Verification items for the finished model (mm, model axes). A direction names the side the tool comes from. Coordinates: 2 decimals unless noted, no trailing zeros. Order: outer loops, then holes, each group sorted by start corner. A loop starts at its lowest first (then second) coordinate and runs counter-clockwise, first axis right, second up. Notation, with made-up numbers: (41, 77.5) -> (81, 77.5) arc R31 ccw to (81, 113.5) -> close; hole circle Ø9 at (2.25, 0). An arc over 180 degrees is marked (long way). Use CSV: the item, a comma, the result in double quotes. Start each with the question number.
1) Tool access check on faces 1 (the flat face through (-24, -34, 0)), 2 (the flat face through (-41.776, -19, -10)), 3 (the flat face through (-27.565, -34, -10)), 4 (the flat face through (-33.537, -42, -10)). Record the directions out of +Z, -Z, +X, -X, +Y, -Y that give a thin tool (end or side, any length) a straight path to the whole face; none if there is none.
2) Release check for a two-part mould opening along Z. For faces 5 (the flat face through (-29, -20, 3.175)), 6 (the flat face through (-29, -20, -23.495)), 7 (the flat face through (-31.339, -34, -10)) record: released by +Z, released by -Z, zero draft, split by the parting line, or undercut.
3) Sectioned sample at D-D on y = -29.5. Record the boundary of the cut face in (x, z) (3 decimals), then the cut area to 3 significant figures.
4) Sectioned sample at A-A on x = -37. Record the boundary of the cut face in (y, z) (3 decimals), then the cut area to 3 significant figures.
5) Sectioned sample at C-C on y = -14. Record the boundary of the cut face in (x, z) (3 decimals).
6) Sectioned sample at B-B on z = -19.5. Record the boundary of the cut face in (x, y).
7) Scan lines: line 1 along Z through (x, y) = (-21, -27) (3 decimals); line 2 along X through (y, z) = (-36.5, -4.25); line 3 along Y through (x, z) = (-1, -12). Record each from-to range of solid material in increasing order.
8) Go/stop test with flat-tipped pins: pin 1 (1.6 mm diameter, centred on x = 4, y = -42.5, fed in from -Z); pin 2 (12 mm diameter, centred on y = -26.5, z = -16, fed in from +X); pin 3 (10 mm diameter, centred on x = -8, z = -9.5, fed in from +Y). Record where each tip stops, or that it passes through.
from build123d import *

# Parameters (mm, degrees)
BOSS_EXTRUDE1_DEPTH = 3.175
SKETCH2_W           = 13.335000012
SKETCH2_H           = 49.21889014
SKETCH2_R           = 1.75
BOSS_EXTRUDE2_DEPTH = 3.175
SKETCH3_W           = 46.34698368
SKETCH3_H           = 3.175
BOSS_EXTRUDE3_DEPTH = 10.160000012
SKETCH4_R           = 1.75
SKETCH4_R_2         = 3.05
CUT_EXTRUDE1_DEPTH  = 8.255
SKETCH5_W           = 3.773247043
SKETCH5_H           = 20.320000025
BOSS_EXTRUDE4_DEPTH = 12.954
SKETCH6_W           = 34.699402295
SKETCH6_H           = 0.254
CUT_EXTRUDE2_DEPTH  = 33.02


with BuildPart() as part:
    # Sketch1 → Boss-Extrude1 (new body)
    with BuildSketch(Plane.XY):
        Polygon((-22.541561274, 5.323288391), (-8.422284226, -43.895601749), (-38.601131181, -43.895601749), (-38.601131181, 5.323288391), align=None)
    extrude(amount=BOSS_EXTRUDE1_DEPTH)

    # Sketch2 → Boss-Extrude2 (add)
    with BuildSketch(Plane.ZY.offset(38.601131181)):
        with Locations((-3.492500006, -19.286156679)):
            Rectangle(SKETCH2_W, SKETCH2_H)
        with Locations(Location((-5.139541866, -3.179625598, 0), (0, 0, 270))):
            Circle(SKETCH2_R, mode=Mode.SUBTRACT)
        with Locations(Location((-5.139541866, -13.22054189, 0), (0, 0, 270))):
            Circle(SKETCH2_R, mode=Mode.SUBTRACT)
    extrude(amount=BOSS_EXTRUDE2_DEPTH)

    # Sketch3 → Boss-Extrude3 (add)
    with BuildSketch(Plane(origin=(0, 0, 0), x_dir=(-1, 0, 0), z_dir=(0, 0, -1))):
        with Locations((10.363026284, -42.308101749)):
            Rectangle(SKETCH3_W, SKETCH3_H)
    extrude(amount=BOSS_EXTRUDE3_DEPTH)

    # Sketch4 → Cut-Extrude1 (cut)
    with BuildSketch(Plane(origin=(0, -40.720601749, 0), x_dir=(1, 0, 0), z_dir=(0, 1, 0))):
        with Locations(Location((-3.706673055, 5.129541844, 0), (0, 0, 270))):
            Circle(SKETCH4_R)
        with Locations(Location((-23.788505641, 5.129541844, 0), (0, 0, 270))):
            Circle(SKETCH4_R)
        with Locations((6.334243237, 15.170458137)):
            Circle(SKETCH4_R)
        with Locations((-8.727131202, 10.149999991)):
            Circle(SKETCH4_R_2)
        with Locations(Location((6.334243237, 5.129541844, 0), (0, 0, 270))):
            Circle(SKETCH4_R)
        with Locations(Location((-13.747589348, 5.129541844, 0), (0, 0, 270))):
            Circle(SKETCH4_R)
        with Locations((-23.788505641, 15.170458137)):
            Circle(SKETCH4_R)
        with Locations((-3.706673055, 15.170458137)):
            Circle(SKETCH4_R)
        with Locations((-13.747589348, 15.170458137)):
            Circle(SKETCH4_R)
    extrude(amount=-CUT_EXTRUDE1_DEPTH, mode=Mode.SUBTRACT)

    # Mirror3: part across plane


with BuildPart() as part_1:
    add(part.part)
    add(part.part.mirror(Plane(origin=(-41.776131181, 5.323288391, -10.160000012), x_dir=(1, 0, 0), z_dir=(0, 0, 1))))

    # Sketch5 → Boss-Extrude4 (add)
    with BuildSketch(Plane(origin=(0, -40.720601749, 0), x_dir=(1, 0, 0), z_dir=(0, 1, 0))):
        with Locations((-29.452107965, 10.160000013)):
            Rectangle(SKETCH5_W, SKETCH5_H)
    extrude(amount=BOSS_EXTRUDE4_DEPTH)

    # Sketch6 → Cut-Extrude2 (cut)
    with BuildSketch(Plane(origin=(0, 5.323288391, 0), x_dir=(1, 0, 0), z_dir=(0, 1, 0))):
        with Locations((-21.251430034, 20.447000025)):
            Rectangle(SKETCH6_W, SKETCH6_H)
        with Locations((-21.251430034, -0.127)):
            Rectangle(SKETCH6_W, SKETCH6_H)
    extrude(amount=-CUT_EXTRUDE2_DEPTH, mode=Mode.SUBTRACT)


solid = part_1.part
Answers follow:
1,face 1,"+Y"
1,face 2,"+Z, -Z, -X, +Y, -Y"
1,face 3,"+X, +Y"
1,face 4,"+Y, -Y"
2,face 5,"released by +Z"
2,face 6,"released by -Z"
2,face 7,"undercut"
3,outline,"(-41.776, -23.495) -> (-12.552, -23.495) -> (-12.552, -20.32) -> (-27.565, -20.32) -> (-27.565, 0) -> (-12.552, 0) -> (-12.552, 3.175) -> (-41.776, 3.175) -> close; hole (-38.601, -20.32) -> (-31.339, -20.32) -> (-31.339, 0) -> (-38.601, 0) -> close"
3,area,"327 mm²"
4,outline,"(-43.896, -23.495) -> (5.323, -23.495) -> (5.323, -20.574) -> (-27.697, -20.574) -> (-27.697, -20.32) -> (-43.896, -20.32) -> close; (-43.896, 0) -> (-27.697, 0) -> (-27.697, 0.254) -> (5.323, 0.254) -> (5.323, 3.175) -> (-43.896, 3.175) -> close"
4,area,"296 mm²"
5,outline,"(-41.776, -23.495) -> (-16.998, -23.495) -> (-16.998, -20.574) -> (-38.601, -20.574) -> (-38.601, -16.747) -> (-41.776, -16.747) -> close; (-41.776, -13.614) -> (-38.601, -13.614) -> (-38.601, -6.706) -> (-41.776, -6.706) -> close; (-41.776, -3.573) -> (-38.601, -3.573) -> (-38.601, 0.254) -> (-16.998, 0.254) -> (-16.998, 3.175) -> (-41.776, 3.175) -> close"
6,outline,"(-41.78, -43.9) -> (-38.6, -43.9) -> (-38.6, 5.32) -> (-41.78, 5.32) -> close; (-33.54, -43.9) -> (12.81, -43.9) -> (12.81, -40.72) -> (-27.57, -40.72) -> (-27.57, -27.77) -> (-31.34, -27.77) -> (-31.34, -40.72) -> (-33.54, -40.72) -> close"
7,line 1,"z = -23.495 to -20.574, 0.254 to 3.175"
7,line 2,"x = -41.78 to -38.6, -31.34 to -27.57"
7,line 3,"y = -43.9 to -40.72"
8,pin 1,"stops at z = -20.32"
8,pin 2,"stops at x = -12.22"
8,pin 3,"stops at y = -40.72"
